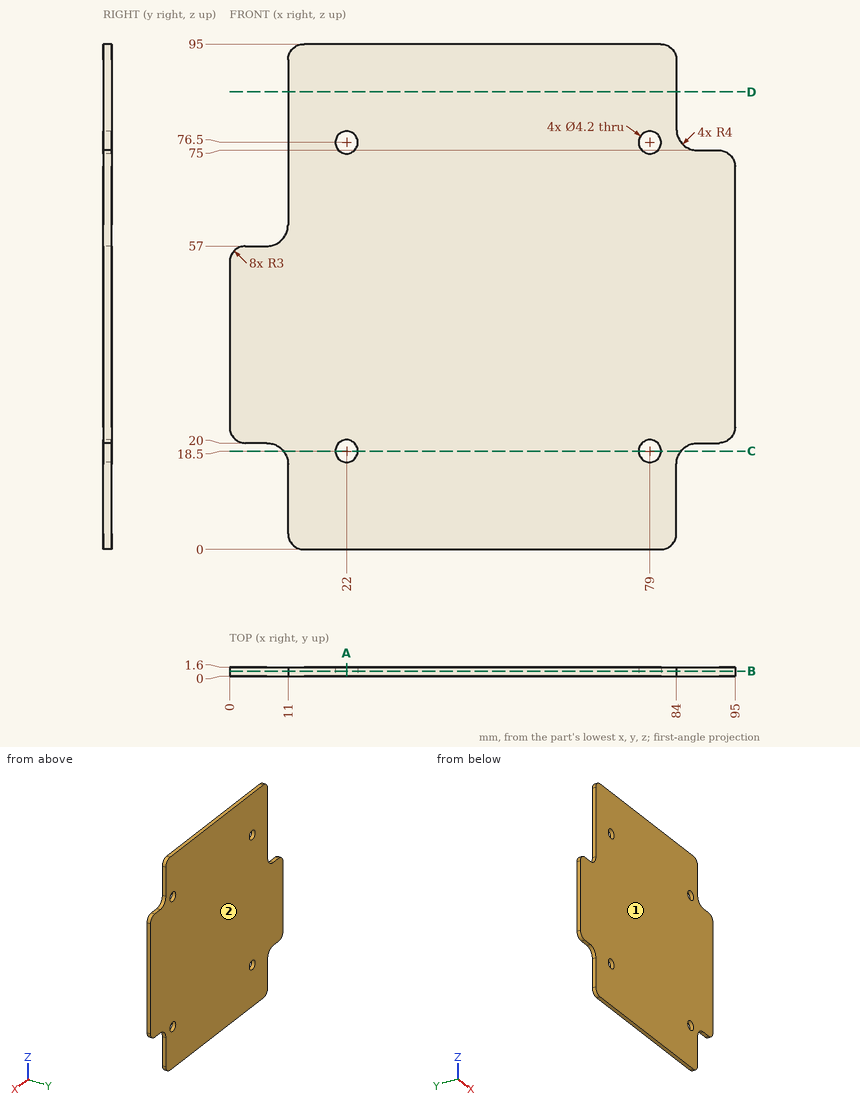
The drawing under review shows one solid part. Ordinate dimensions are in mm from its lowest x, y, z. Give positions to 0.01 mm unless a question says otherwise; leave off trailing zeros. Write each loop counter-clockwise with the first axis right and the second up, starting at its lowest first coordinate (ties: lowest second). Pieces come first, ordered by that corner, then holes. Notation, with made-up numbers: (68, 60.25) -> (123, 60.25) arc R16 ccw to (123, 81.25) -> close; hole circle Ø1 at (69, 85). An arc over 180 degrees is marked (long way). Answer in a Markdown table with one row per item.
(1) To check wall thickness, follow probe 1 along Z at (x, y) = (79, 0.7); probe 2 along X at (y, z) = (0.65, 18.5); probe 3 along X at (y, z) = (0.9, 76.5). State the ranges of each line that lie inside material, in increasing order.
Results:
| item | result |
|---|---|
| probe 1 | 0 to 16.4, 20.6 to 74.4, 78.6 to 95 |
| probe 2 | 10.12 to 19.9, 24.1 to 76.9, 81.1 to 84.88 |
| probe 3 | 11 to 19.9, 24.1 to 76.9, 81.1 to 84.88 |
(2) Consider section C-C (z = 18.5). State the section outline as (x, y) points.
Results:
| item | result |
|---|---|
| outline | (10.12, 0) -> (19.9, 0) -> (19.9, 1.6) -> (10.12, 1.6) -> close; (24.1, 0) -> (76.9, 0) -> (76.9, 1.6) -> (24.1, 1.6) -> close; (81.1, 0) -> (84.88, 0) -> (84.88, 1.6) -> (81.1, 1.6) -> close |
(3) Consider section D-D (z = 86). State the section outline as (x, y) points.
Results:
| item | result |
|---|---|
| outline | (11, 0) -> (84, 0) -> (84, 1.6) -> (11, 1.6) -> close |
(4) Consider section B-B (y = 0.9). State the section outline as (x, z) points, then the cut area to 3 significant figures.
Results:
| item | result |
|---|---|
| outline | (0, 23) arc R3 ccw to (3, 20) -> (7, 20) arc R4 cw to (11, 16) -> (11, 3) arc R3 ccw to (14, 0) -> (81, 0) arc R3 ccw to (84, 3) -> (84, 16) arc R4 cw to (88, 20) -> (92, 20) arc R3 ccw to (95, 23) -> (95, 72) arc R3 ccw to (92, 75) -> (88, 75) arc R4 cw to (84, 79) -> (84, 92) arc R3 ccw to (81, 95) -> (14, 95) arc R3 ccw to (11, 92) -> (11, 61) arc R4 cw to (7, 57) -> (3, 57) arc R3 ccw to (0, 54) -> close; hole circle Ø4.2 at (22, 18.5); hole circle Ø4.2 at (22, 76.5); hole circle Ø4.2 at (79, 18.5); hole circle Ø4.2 at (79, 76.5) |
| area | 7,890 mm2 |
(5) Mouldability with a two-part tool opening along Y and no side actions: class the marked faces 1 and 2 as +Y half, -Y half, draft (parallel to the pull), parting line (faces both ways), or undercut.
Results:
| item | result |
|---|---|
| face 1 | -Y half |
| face 2 | +Y half |
(6) Consider section A-A (x = 22). State the section outline as (y, z) points.
Results:
| item | result |
|---|---|
| outline | (0, 0) -> (1.6, 0) -> (1.6, 16.4) -> (0, 16.4) -> close; (0, 20.6) -> (1.6, 20.6) -> (1.6, 74.4) -> (0, 74.4) -> close; (0, 78.6) -> (1.6, 78.6) -> (1.6, 95) -> (0, 95) -> close |
(7) Clearance check with flat-ended pins moving along their axes: pin 1 (0.5 mm diameter, centred on x = 4, y = 1, fed in from +Z); pin 2 (4 mm diameter, centred on x = 18.5, z = 73.5, fed in from -Y); pin 3 (2.5 mm diameter, centred on x = 22, z = 18.5, fed in from -Y); pin 4 (0.8 mm diameter, centred on x = 4.5, y = 1, fed in from -Z). State where each tip first meets the part, or that it passes through.
Results:
| item | result |
|---|---|
| pin 1 | z = 57 |
| pin 2 | y = 0 |
| pin 3 | through |
| pin 4 | z = 20 |
